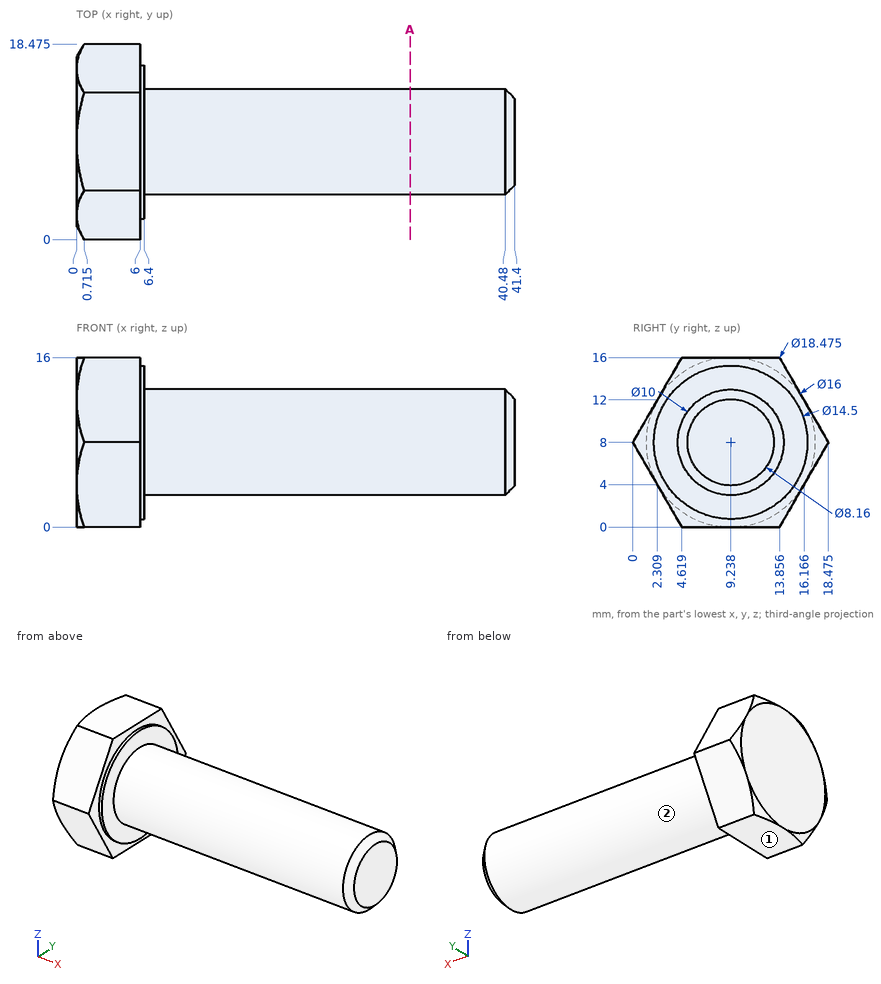
Input: dimensioned drawing with shaded views. Units: mm. Origin: part minimum x, y, z. A direction names the side the tool comes from. Round coordinates to 2 decimals unless told otherwise and drop trailing zeros. Loops run counter-clockwise (first coordinate to the right, second up) from the corner with the lowest first, then second, coordinate; pieces in that order, holes last.
1) Pin query (flat end, axial travel): pin 1 (4 mm diameter, centred on x = 12, z = 3, fed in from +Y); pin 2 (1 mm diameter, centred on x = 6, y = 14.5, fed in from -Z); pin 3 (4 mm diameter, centred on x = 27.5, z = 7, fed in from -Y). Return the tip coordinate at first contact, or that it passes through.
Ans:
pin 1: stops at y = 13.24
pin 2: stops at z = 0.25
pin 3: stops at y = 4.24
2) Set-up query: the marked faces 1 and 2. Return all of +Z, -Z, +X, -X, +Y, -Y with unobstructed straight access to the full face (end or side cutting, diameter ignored); none if empty.
Ans:
face 1: -Z, +X, -X, +Y, -Y
face 2: +X
3) Material intervals for line 1 (X direction, y = 12.75, z = 3); line 2 (X direction, y = 17, z = 9); line 3 (Y direction, x = 27.5, z = 11.25) (1 decimal), sorted ascending.
Ans:
line 1: x = 0 to 6.4
line 2: x = 0 to 6
line 3: y = 5.4 to 13
4) Section query A-A on x = 31.5. Return the cut outline in (y, z).
Ans:
outline: circle Ø10 at (9.24, 8)
